from build123d import *

# Parameters (mm, degrees)
ESQUISSE1_W             = 88
ESQUISSE1_H             = 42
BOSS_EXTRU_1_DEPTH      = 20
ESQUISSE2_W             = 82.4
ESQUISSE2_H             = 36.4
ENL_V_MAT_EXTRU_1_DEPTH = 17
ESQUISSE3_W             = 14
ESQUISSE3_H             = 15.4
ESQUISSE3_W_2           = 15
ESQUISSE3_H_2           = 24
ESQUISSE3_W_3           = 8.4
ESQUISSE3_H_3           = 11.4
ENL_V_MAT_EXTRU_3_DEPTH = 53


with BuildPart() as part:
    # Esquisse1 → Boss.-Extru.1 (new body)
    with BuildSketch(Plane(origin=(0, 0, 0), x_dir=(1, 0, 0), z_dir=(0, 1, 0))):
        with Locations((-25.603062664, -21.590445487)):
            Rectangle(ESQUISSE1_W, ESQUISSE1_H)
    extrude(amount=BOSS_EXTRU_1_DEPTH)

    # Esquisse2 → Enlèv. mat.-Extru.1 (cut)
    with BuildSketch(Plane(origin=(0, 0, 0), x_dir=(1, 0, 0), z_dir=(0, 1, 0))):
        with Locations((-25.603062664, -21.590445487)):
            Rectangle(ESQUISSE2_W, ESQUISSE2_H)
    extrude(amount=ENL_V_MAT_EXTRU_1_DEPTH, mode=Mode.SUBTRACT)

    # Esquisse3 → Enlèv. mat.-Extru.3 (cut)
    with BuildSketch(Plane(origin=(0, 0, 0), x_dir=(1, 0, 0), z_dir=(0, 1, 0))):
        with Locations((5.596937336, -24.090445487)):
            Rectangle(ESQUISSE3_W, ESQUISSE3_H)
        with Locations((-20.403062664, -24.090445487)):
            Rectangle(ESQUISSE3_W, ESQUISSE3_H)
        with Locations((-46.903062664, -28.390445487)):
            Rectangle(ESQUISSE3_W_2, ESQUISSE3_H_2)
        with Locations((-60.603062664, -13.090445487)):
            Rectangle(ESQUISSE3_W_3, ESQUISSE3_H_3)
    extrude(amount=ENL_V_MAT_EXTRU_3_DEPTH, mode=Mode.SUBTRACT)


solid = part.part
Design review of the part built by this model. Coordinates are the model's own, in mm. A direction names the side the tool comes from. Round coordinates to 2 decimals unless told otherwise and drop trailing zeros. Write each loop counter-clockwise with the first axis right and the second up, starting at its lowest first coordinate (ties: lowest second). Pieces come first, ordered by that corner, then holes. Notation, with made-up numbers: (-8, 57.25) -> (30, 57.25) arc R27 cw to (30, 96.25) -> close; hole circle Ø2 at (38, -38.75). An arc over 180 degrees is marked (long way). One line per item, written item: value. Start each with the question number.
Q1. Tool access review of faces 4 (the face through (-26, 8, 3.39)), 5 (the face through (-26, 0, 3)), 6 (the face through (-39.403, 17.4, 30.2)): name each direction out of +Z, -Z, +X, -X, +Y, -Y from which nothing blocks a thin tool from reaching the whole face with its end or side.
Q2. Add section B-B (y = 8.25). Give the boundary of the cut face in (x, z), then the cut area to 3 significant figures.
Q3. The part is to be moulded in two halves that separate along Z. For faces 1 (the face through (-26, 10, 0.59)), 2 (the face through (-26, 20, 12)), 3 (the face through (-21, 18, 16.39)), say which applies: pulls with the +Z half, pulls with the -Z half, needs draft (parallel to the pull), parting line crosses it, or undercut.
Q4. Insertion check: P1, Ø18, axis at x = -22, z = 18.5, coming from the -Y side. The pin has a flat end and moves straight along its axis. Give the tip position at first contact, or say it passes through.
Q5. Add section D-D (z = 28.5). Give the boundary of the cut face in (x, y).
Q6. To check wall thickness, follow probe 1 along Z at (x, y) = (-37.5, 16.5); probe 2 along Z at (x, y) = (-50.5, 14.5); probe 3 along X at (y, z) = (4.25, 25). State the ranges of each line that lie inside material, in increasing order.
Q7. Add section C-C (z = 8.5). Give the boundary of the cut face in (x, y), then the cut area to 3 significant figures.
Q8. Add section A-A (x = -63.5). Give the boundary of the cut face in (y, z), then the cut area to 3 significant figures.
Response:
1. face 4: -Y
1. face 5: +Z, -Z, +X, -X, -Y
1. face 6: +Y, -Y
2. outline: (-69.6, 0.59) -> (18.4, 0.59) -> (18.4, 42.59) -> (-69.6, 42.59) -> close; hole (-66.8, 3.39) -> (15.6, 3.39) -> (15.6, 39.79) -> (-39.4, 39.79) -> (-39.4, 40.39) -> (-54.4, 40.39) -> (-54.4, 39.79) -> (-66.8, 39.79) -> close
2. area: 688 mm^2
3. face 1: pulls with the -Z half
3. face 2: needs draft
3. face 3: undercut
4. P1: stops at y = 17
5. outline: (-69.6, 0) -> (-66.8, 0) -> (-66.8, 17) -> (-54.4, 17) -> (-54.4, 20) -> (-69.6, 20) -> close; (-39.4, 17) -> (-27.4, 17) -> (-27.4, 20) -> (-39.4, 20) -> close; (-13.4, 17) -> (-1.4, 17) -> (-1.4, 20) -> (-13.4, 20) -> close; (12.6, 17) -> (15.6, 17) -> (15.6, 0) -> (18.4, 0) -> (18.4, 20) -> (12.6, 20) -> close
6. probe 1: z = 0.59 to 3.39, 39.79 to 42.59
6. probe 2: z = 0.59 to 3.39, 40.39 to 42.59
6. probe 3: x = -69.6 to -66.8, 15.6 to 18.4
7. outline: (-69.6, 0) -> (-66.8, 0) -> (-66.8, 17) -> (-64.8, 17) -> (-64.8, 20) -> (-69.6, 20) -> close; (-56.4, 17) -> (15.6, 17) -> (15.6, 0) -> (18.4, 0) -> (18.4, 20) -> (-56.4, 20) -> close
7. area: 334 mm^2
8. outline: (0, 0.59) -> (20, 0.59) -> (20, 7.39) -> (17, 7.39) -> (17, 3.39) -> (0, 3.39) -> close; (0, 39.79) -> (17, 39.79) -> (17, 18.79) -> (20, 18.79) -> (20, 42.59) -> (0, 42.59) -> close
8. area: 187 mm^2
